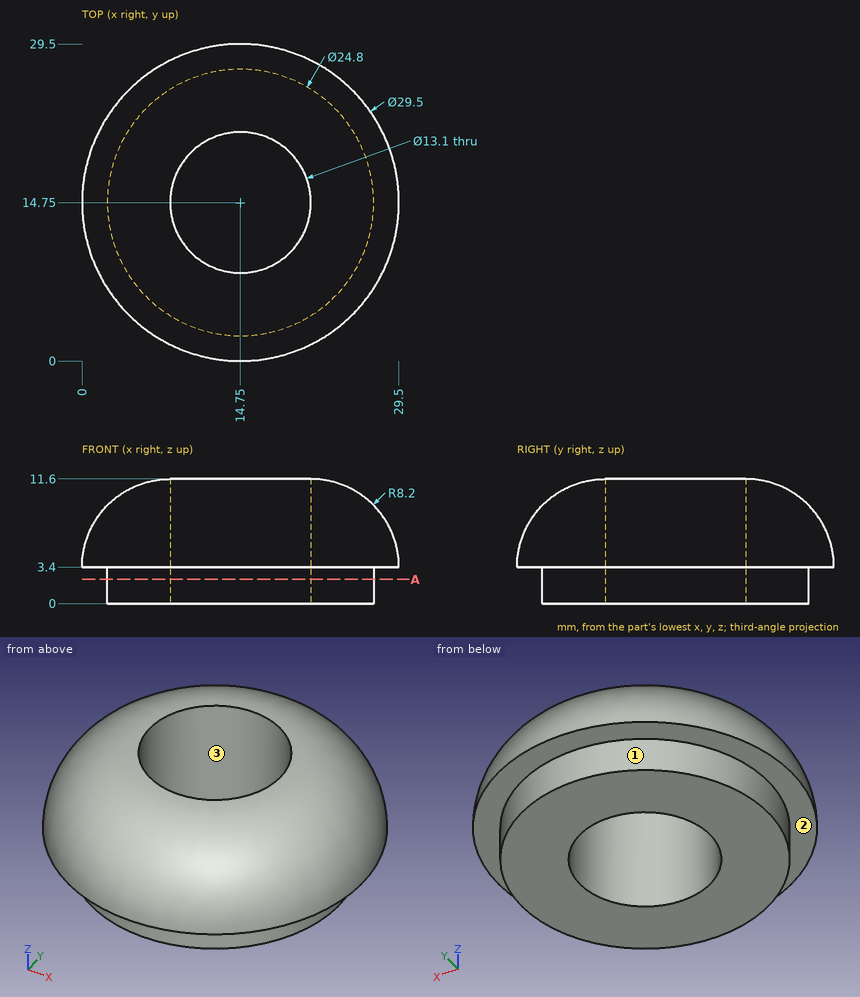
Study the drawing (mm; zero at the part's minimum x, y, z) and answer. Round coordinates to 2 decimals unless told otherwise and drop trailing zeros. Write each loop counter-clockwise with the first axis right and the second up, starting at its lowest first coordinate (ties: lowest second). Pieces come first, ordered by that corner, then holes.
1) Given pin 1 Ø4 at (y, z) = (26.5, 7.5) entering from +X; pin 2 Ø3 at (y, z) = (20.5, 8) entering from +X; pin 3 Ø1.5 at (x, z) = (16.5, 10) entering from -Y, each flat-ended and moving along its own axis, determine where each tip first touches the part or whether it passes through.
2) The mould has two halves that part along Y. Classify the marked faces 1, 2 and 3: pulls with the +Y half, pulls with the -Y half, needs draft (parallel to the pull), parting line crosses it, or undercut.
3) A cutting plane is placed at A-A (z = 2.25). Give the vertices of the cut face in (x, y), plus the area to 3 significant figures.
4) Straight lines are drawn through the part: line 1 (Y direction, x = 14.75, z = 2.75); line 2 (Y direction, x = 14.75, z = 6.5); line 3 (X direction, y = 18, z = 7.25). For each, find the intervals that lie inside material, in ascending order.
Completed:
1. pin 1: stops at x = 24.73
1. pin 2: stops at x = 27.9
1. pin 3: stops at y = 2.57
2. face 1: parting line crosses it
2. face 2: needs draft
2. face 3: undercut
3. outline: circle Ø24.8 at (14.75, 14.75); hole circle Ø13.1 at (14.75, 14.75)
3. area: 348 mm2
4. line 1: y = 2.35 to 8.2, 21.3 to 27.15
4. line 2: y = 0.61 to 8.2, 21.3 to 28.89
4. line 3: x = 1.35 to 9.06, 20.44 to 28.15
